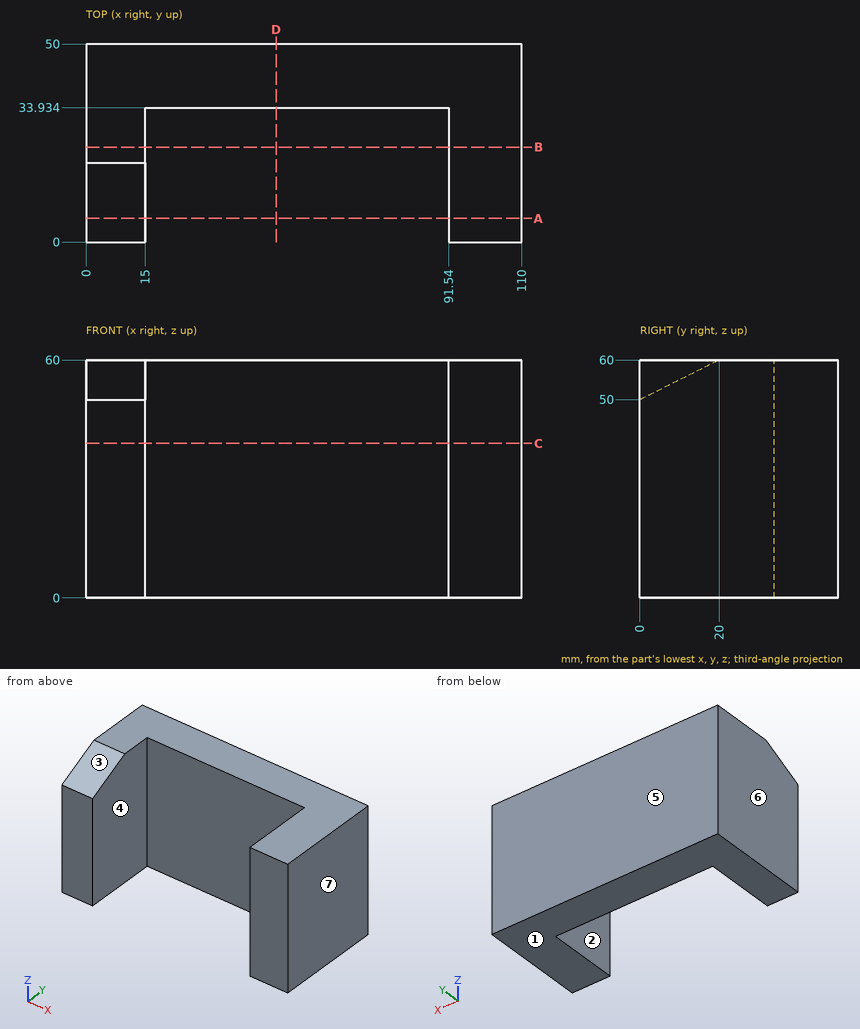
Check sheet for the drawn part. Datum: minimum x, y, z corner. Units: mm. A direction names the side the tool comes from. Coordinates: 2 decimals unless noted, no trailing zeros. Loops run counter-clockwise (first coordinate to the right, second up) from the corner with the lowest first, then second, coordinate; pieces in that order, holes last. Notation, with made-up numbers: (-10, -1) -> (23, -1) arc R18 ccw to (23, 31) -> close; hole circle Ø9 at (-20.75, -12.5). An arc over 180 degrees is marked (long way). Write each question's results on one line, items separated by ' | '.
Item 1: Mould release check, pull along X, two halves, no side actions. Record for the marked faces 4, 5, 6 and 7: +X half, -X half, draft (parallel to the pull), parting line (faces both ways), or undercut.
Found:
face 4: undercut | face 5: draft | face 6: -X half | face 7: +X half
Item 2: Material ranges on L1, parallel to X at y = 4, z = 40.5; L2, parallel to Y at x = 88.5, z = 44.5; L3, parallel to Z at x = 13, y = 3, recorded low to high.
Found:
L1: x = 0 to 15, 91.54 to 110 | L2: y = 33.93 to 50 | L3: z = 0 to 51.5
Item 3: Gauge pin test, flat end, axial feed: pin 1 (4 mm diameter, centred on x = 36.5, z = 8.5, fed in from -Y). Record the tip position at first contact, or that the pin passes through.
Found:
pin 1: stops at y = 33.93
Item 4: Section check C-C, the plane z = 39. Enter the section's corners in (x, y), plus the area to 3 significant figures.
Found:
outline: (0, 0) -> (15, 0) -> (15, 33.93) -> (91.54, 33.93) -> (91.54, 0) -> (110, 0) -> (110, 50) -> (0, 50) -> close | area: 2,900 mm2
Item 5: Tool access check on the marked faces 1, 2 and 3. Record the directions out of +Z, -Z, +X, -X, +Y, -Y that give a thin tool (end or side, any length) a straight path to the whole face; none if there is none.
Found:
face 1: -Z, +X, -X, +Y, -Y | face 2: +Z, -Z, -Y | face 3: +Z, -X, -Y
Item 6: Section check B-B, the plane y = 24. Enter the section's corners in (x, z), plus the area to 3 significant figures.
Found:
outline: (0, 0) -> (15, 0) -> (15, 60) -> (0, 60) -> close; (91.54, 0) -> (110, 0) -> (110, 60) -> (91.54, 60) -> close | area: 2,010 mm2
Item 7: Section check A-A, the plane y = 6. Enter the section's corners in (x, z), plus the area to 3 significant figures.
Found:
outline: (0, 0) -> (15, 0) -> (15, 53) -> (0, 53) -> close; (91.54, 0) -> (110, 0) -> (110, 60) -> (91.54, 60) -> close | area: 1,900 mm2
Item 8: Section check D-D, the plane x = 48. Enter the section's corners in (y, z), plus the area to 3 significant figures.
Found:
outline: (33.93, 0) -> (50, 0) -> (50, 60) -> (33.93, 60) -> close | area: 964 mm2
